from build123d import *

# Parameters (mm, degrees)
SKETCH1_R           = 17
SKETCH1_R_2         = 7
BOSS_EXTRUDE1_DEPTH = 50
SKETCH2_R           = 2.5
CUT_EXTRUDE1_DEPTH  = 56.479726027
SKETCH3_R           = 2.5
CUT_EXTRUDE2_DEPTH  = 56.479726178


with BuildPart() as part:
    # Sketch1 → Boss-Extrude1 (new body)
    with BuildSketch(Plane(origin=(0, 0, 0), x_dir=(1, 0, 0), z_dir=(0, 1, 0))):
        with Locations(Location((0, 0, 0), (0, 0, 270))):
            Circle(SKETCH1_R)
        with Locations(Location((0, 0, 0), (0, 0, 270))):
            Circle(SKETCH1_R_2, mode=Mode.SUBTRACT)
    extrude(amount=BOSS_EXTRUDE1_DEPTH)

    # Sketch2 → Cut-Extrude1 (cut, through all)
    with BuildSketch(Plane.XY):
        with Locations(Location((0, 44, 0), (0, 0, 90))):
            Circle(SKETCH2_R)
        with Locations(Location((0, 6, 0), (0, 0, 90))):
            Circle(SKETCH2_R)
    extrude(amount=-CUT_EXTRUDE1_DEPTH, mode=Mode.SUBTRACT)

    # Sketch3 → Cut-Extrude2 (cut, through all)
    with BuildSketch(Plane(origin=(0, 0, 0), x_dir=(0, 0, -1), z_dir=(1, 0, 0))):
        with Locations((0, 44)):
            Circle(SKETCH3_R)
        with Locations((0, 6)):
            Circle(SKETCH3_R)
    extrude(amount=-CUT_EXTRUDE2_DEPTH, mode=Mode.SUBTRACT)


solid = part.part
Read the model definition and answer for the solid it produces. Units are mm, in the model's axes. A direction names the side the tool comes from. Round coordinates to 2 decimals unless told otherwise and drop trailing zeros. Order: outer loops, then holes, each group sorted by start corner. A loop starts at its lowest first (then second) coordinate and runs counter-clockwise, first axis right, second up. Notation, with made-up numbers: (43.25, 10) - (75.25, 10) arc R26 cw to (75.25, 29) - close; hole circle Ø3 at (9, 33). An arc over 180 degrees is marked (long way). Use one line per item in the form item = value. Start each with the question number.
(1) The part is cut by section A-A (z = 0). Give the vertices of the cut face in (x, y), then the cut area to 3 significant figures.
(2) Find the intervals of material crossed by line 1 along Y through (x, z) = (-13, 0); line 2 along X through (y, z) = (30.5, 0); line 3 along Z through (x, y) = (-13, 44), in increasing order. Write a range as from..to.
(3) The part is cut by section D-D (x = 5). Give the vertices of the cut face in (y, z).
(4) The part is cut by section B-B (x = 0). Give the vertices of the cut face in (y, z).
(5) For faces 1 (the face through (0.96, 46.31, -11.7)), 2 (the face through (-11.7, 8.48, 0.33)), 3 (the face through (0.2, 0, 7.3)), determine the directions among +Z, -Z, +X, -X, +Y, -Y from which every point of the face is accessible in a straight line to the end or side of a thin tool.
(6) Determine the mould class of faces 4 (the face through (-11.7, 41.56, 0.54)), 5 (the face through (0.2, 50, 7.3)), 6 (the face through (5.106, 24.65, 16.215)) for opening direction Z: +Z half, -Z half, draft (parallel to the pull), parting line (faces both ways), or undercut.
(7) The part is cut by section C-C (y = 44). Give the vertices of the cut face in (x, z).
(8) Flat-ended cylindrical pins translate along their axes: pin 1 Ø1 at (x, y) = (8.5, 39) entering from -Z; pin 2 Ø4 at (x, y) = (-6.5, 14.5) entering from -Z; pin 3 Ø6 at (y, z) = (30, 4.5) entering from +X. Find the tip coordinate at first contact, or state that the pin passes through.
Checked values:
q1.outline = (-17, 0) - (-7, 0) - (-7, 3.5) - (-17, 3.5) - close; (-17, 8.5) - (-7, 8.5) - (-7, 41.5) - (-17, 41.5) - close; (-17, 46.5) - (-7, 46.5) - (-7, 50) - (-17, 50) - close; (7, 0) - (17, 0) - (17, 50) - (7, 50) - close
q1.area = 900 mm^2
q2.line_1 = 0..3.5, 8.5..41.5, 46.5..50
q2.line_2 = -17..-7, 7..17
q2.line_3 = -10.95..-2.5, 2.5..10.95
q3.outline = (0, -16.25) - (50, -16.25) - (50, -4.9) - (0, -4.9) - close; (0, 4.9) - (50, 4.9) - (50, 16.25) - (0, 16.25) - close
q4.outline = (0, -17) - (3.5, -17) - (3.5, -7) - (0, -7) - close; (0, 7) - (50, 7) - (50, 17) - (0, 17) - close; (8.5, -17) - (41.5, -17) - (41.5, -7) - (8.5, -7) - close; (46.5, -17) - (50, -17) - (50, -7) - (46.5, -7) - close
q5.face_1 = -Z
q5.face_2 = -X
q5.face_3 = +Z, -Z, +X, -X, -Y
q6.face_4 = undercut
q6.face_5 = draft
q6.face_6 = parting line
q7.outline = (-16.82, -2.5) arc R17 ccw to (-2.5, -16.82) - (-2.5, -6.54) arc R7 cw to (-6.54, -2.5) - close; (-16.82, 2.5) - (-6.54, 2.5) arc R7 cw (long way) to (2.5, -6.54) - (2.5, -16.82) arc R17 ccw (long way) to start
q8.pin_1 = -15
q8.pin_2 = -16.39
q8.pin_3 = 16.93
